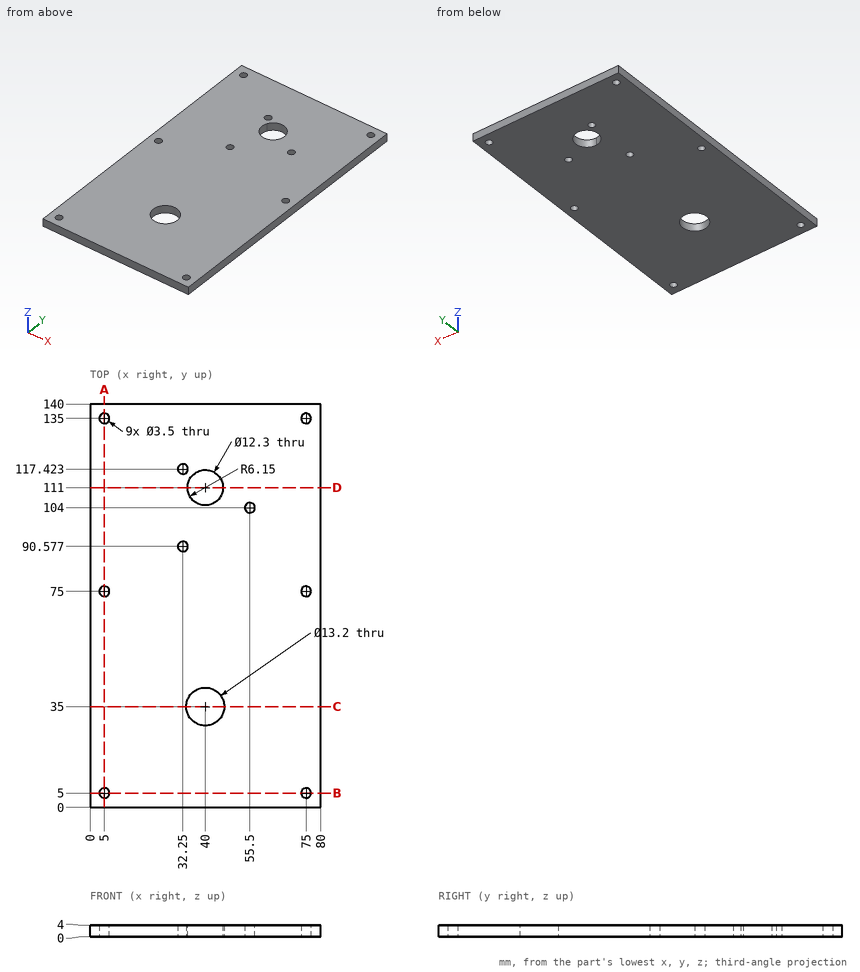
Part print with two shaded views. Sizes in mm from the minimum x, y, z corner. Coordinates: 2 decimals unless noted, no trailing zeros. Order: outer loops, then holes, each group sorted by start corner. A loop starts at its lowest first (then second) coordinate and runs counter-clockwise, first axis right, second up. Notation, with made-up numbers: M 60.25,-39 L 88.25,-39 A18 cw 88.25,-18 Z; hole C 39,68 d10. An arc over 180 degrees is marked long. One line per question, with ' | ' between items. Start each with the question number.
1. Cut at D-D (y = 111). Write the cut outline in (x, z).
2. Cut at C-C (y = 35). Write the cut outline in (x, z).
3. Flat gauge pins, fed straight in: P1, Ø2, axis at x = 75, y = 135, coming from the -Z side; P2, Ø4.5, axis at x = 5, y = 75, coming from the +Z side. Where does each tip first touch, or does it go through?
4. Cut at B-B (y = 5). Write the cut outline in (x, z).
5. Cut at A-A (x = 5). Write the cut outline in (y, z), plus the area to 3 significant figures.
6. Wall check: line 1 along Y through (x, z) = (75, 2.5); line 2 along X through (y, z) = (135, 1.5); line 3 along X through (y, z) = (76, 1.15) (1 decimal). Give the ranges that are in metal, low to high. Write a range as [from, to].
The answers:
1) outline: M 0,0 L 33.85,0 L 33.85,4 L 0,4 Z; M 46.15,0 L 80,0 L 80,4 L 46.15,4 Z
2) outline: M 0,0 L 33.4,0 L 33.4,4 L 0,4 Z; M 46.6,0 L 80,0 L 80,4 L 46.6,4 Z
3) P1: passes through | P2: stops at z = 4
4) outline: M 0,0 L 3.25,0 L 3.25,4 L 0,4 Z; M 6.75,0 L 73.25,0 L 73.25,4 L 6.75,4 Z; M 76.75,0 L 80,0 L 80,4 L 76.75,4 Z
5) outline: M 0,0 L 3.25,0 L 3.25,4 L 0,4 Z; M 6.75,0 L 73.25,0 L 73.25,4 L 6.75,4 Z; M 76.75,0 L 133.25,0 L 133.25,4 L 76.75,4 Z; M 136.75,0 L 140,0 L 140,4 L 136.75,4 Z | area: 518 mm2
6) line 1: y = [0, 3.25], [6.75, 73.25], [76.75, 133.25], [136.75, 140] | line 2: x = [0, 3.25], [6.75, 73.25], [76.75, 80] | line 3: x = [0, 3.6], [6.4, 73.6], [76.4, 80]
